Input: part model. Units: mm. Frame: model coordinates. Face numbers are marked on the shaded views. A direction names the side the tool comes from. Coordinates: 2 decimals unless noted, no trailing zeros. Write each loop counter-clockwise with the first axis right and the second up, starting at its lowest first coordinate (ties: lowest second). Pieces come first, ordered by that corner, then holes. Notation, with made-up numbers: (-26, 18.5) - (11, 18.5) arc R14 cw to (11, 45.5) - close; hole circle Ø3 at (-24.75, -27). An arc over 180 degrees is marked (long way). Put each result on its own line as item: value. Start each with the question number.
1. Line query: line 1 (X direction, y = 1.05, z = -11.06); line 2 (Z direction, x = 15.9, y = 0.6); line 3 (Y direction, x = -7, z = -9). Output: solid intervals per line, ascending.
2. Cut plane A-A, the plane z = 0. Return loops of the section in (x, y).
3. Pin query (flat end, axial travel): pin 1 (6.5 mm diameter, centred on x = -19, z = -14.5, fed in from +Y); pin 2 (5.5 mm diameter, centred on x = -17.85, z = 13.01, fed in from -Y); pin 3 (5.5 mm diameter, centred on x = 17.85, z = 13.01, fed in from +Y). Return the tip coordinate at first contact, or that it passes through.
4. Access query for the marked faces 1, 2, 3 and 4. Directions: +Z, -Z, +X, -X, +Y, -Y. A direction counts if a zero-diameter tool reaches every point of the face in a straight line with its end or side. Return the directions, or none.
5. Cut plane C-C, the plane x = 8.5. Return loops of the section in (y, z), and give its area (3 significant figures).
6. Cut plane B-B, the plane y = 5.5. Return loops of the section in (x, z), and give its area (3 significant figures).
from build123d import *

# Parameters (mm, degrees)
CROQUIS1_W              = 41.94
CROQUIS1_H              = 32.26
CROQUIS1_R              = 1.65
CROQUIS1_R_2            = 0.2
SALIENTE_EXTRUIR1_DEPTH = 1.64
CORTAR_EXTRUIR1_START   = -0.1
CROQUIS2_R              = 3.04
CROQUIS2_R_2            = 1.65
CORTAR_EXTRUIR1_DEPTH   = 0.1
REDONDEO2_R             = 3
CROQUIS3_W              = 7.8
CROQUIS3_H              = 10.08
SALIENTE_EXTRUIR2_DEPTH = 6.7


with BuildPart() as part:
    # Croquis1 → Saliente-Extruir1 (new body)
    with BuildSketch(Plane(origin=(0, 0, 0), x_dir=(1, 0, 0), z_dir=(0, 1, 0))):
        Rectangle(CROQUIS1_W, CROQUIS1_H)
        with Locations(Location((-17.85, 13.01, 0), (0, 0, 270))):
            Circle(CROQUIS1_R, mode=Mode.SUBTRACT)
        with Locations(Location((17.85, 13.01, 0), (0, 0, 90))):
            Circle(CROQUIS1_R, mode=Mode.SUBTRACT)
        with Locations(Location((17.85, -13.01, 0), (0, 0, 270))):
            Circle(CROQUIS1_R, mode=Mode.SUBTRACT)
        with Locations(Location((-17.85, -13.01, 0), (0, 0, 90))):
            Circle(CROQUIS1_R, mode=Mode.SUBTRACT)
        with Locations(Location((-15.9, 13.01, 0), (0, 0, 270))):
            Circle(CROQUIS1_R_2, mode=Mode.SUBTRACT)
        with Locations(Location((-16.471141777, 11.631141777, 0), (0, 0, 270))):
            Circle(CROQUIS1_R_2, mode=Mode.SUBTRACT)
        with Locations(Location((-17.85, 11.06, 0), (0, 0, 270))):
            Circle(CROQUIS1_R_2, mode=Mode.SUBTRACT)
        with Locations(Location((-19.228858223, 11.631141777, 0), (0, 0, 270))):
            Circle(CROQUIS1_R_2, mode=Mode.SUBTRACT)
        with Locations(Location((-19.8, 13.01, 0), (0, 0, 270))):
            Circle(CROQUIS1_R_2, mode=Mode.SUBTRACT)
        with Locations(Location((-19.228858223, 14.388858223, 0), (0, 0, 270))):
            Circle(CROQUIS1_R_2, mode=Mode.SUBTRACT)
        with Locations(Location((-17.85, 14.96, 0), (0, 0, 270))):
            Circle(CROQUIS1_R_2, mode=Mode.SUBTRACT)
        with Locations(Location((-16.471141777, 14.388858223, 0), (0, 0, 270))):
            Circle(CROQUIS1_R_2, mode=Mode.SUBTRACT)
        with Locations(Location((19.8, 13.01, 0), (0, 0, 90))):
            Circle(CROQUIS1_R_2, mode=Mode.SUBTRACT)
        with Locations(Location((19.228858223, 14.388858223, 0), (0, 0, 90))):
            Circle(CROQUIS1_R_2, mode=Mode.SUBTRACT)
        with Locations(Location((17.85, 14.96, 0), (0, 0, 90))):
            Circle(CROQUIS1_R_2, mode=Mode.SUBTRACT)
        with Locations(Location((16.471141777, 14.388858223, 0), (0, 0, 90))):
            Circle(CROQUIS1_R_2, mode=Mode.SUBTRACT)
        with Locations(Location((15.9, 13.01, 0), (0, 0, 90))):
            Circle(CROQUIS1_R_2, mode=Mode.SUBTRACT)
        with Locations(Location((16.471141777, 11.631141777, 0), (0, 0, 90))):
            Circle(CROQUIS1_R_2, mode=Mode.SUBTRACT)
        with Locations(Location((19.228858223, 11.631141777, 0), (0, 0, 90))):
            Circle(CROQUIS1_R_2, mode=Mode.SUBTRACT)
        with Locations(Location((17.85, 11.06, 0), (0, 0, 90))):
            Circle(CROQUIS1_R_2, mode=Mode.SUBTRACT)
        with Locations(Location((19.228858223, -11.631141777, 0), (0, 0, 270))):
            Circle(CROQUIS1_R_2, mode=Mode.SUBTRACT)
        with Locations(Location((19.8, -13.01, 0), (0, 0, 270))):
            Circle(CROQUIS1_R_2, mode=Mode.SUBTRACT)
        with Locations(Location((19.228858223, -14.388858223, 0), (0, 0, 270))):
            Circle(CROQUIS1_R_2, mode=Mode.SUBTRACT)
        with Locations(Location((17.85, -14.96, 0), (0, 0, 270))):
            Circle(CROQUIS1_R_2, mode=Mode.SUBTRACT)
        with Locations(Location((16.471141777, -14.388858223, 0), (0, 0, 270))):
            Circle(CROQUIS1_R_2, mode=Mode.SUBTRACT)
        with Locations(Location((15.9, -13.01, 0), (0, 0, 270))):
            Circle(CROQUIS1_R_2, mode=Mode.SUBTRACT)
        with Locations(Location((17.85, -11.06, 0), (0, 0, 270))):
            Circle(CROQUIS1_R_2, mode=Mode.SUBTRACT)
        with Locations(Location((16.471141777, -11.631141777, 0), (0, 0, 270))):
            Circle(CROQUIS1_R_2, mode=Mode.SUBTRACT)
        with Locations(Location((-19.228858223, -14.388858223, 0), (0, 0, 90))):
            Circle(CROQUIS1_R_2, mode=Mode.SUBTRACT)
        with Locations(Location((-17.85, -14.96, 0), (0, 0, 90))):
            Circle(CROQUIS1_R_2, mode=Mode.SUBTRACT)
        with Locations(Location((-16.471141777, -14.388858223, 0), (0, 0, 90))):
            Circle(CROQUIS1_R_2, mode=Mode.SUBTRACT)
        with Locations(Location((-15.9, -13.01, 0), (0, 0, 90))):
            Circle(CROQUIS1_R_2, mode=Mode.SUBTRACT)
        with Locations(Location((-19.8, -13.01, 0), (0, 0, 90))):
            Circle(CROQUIS1_R_2, mode=Mode.SUBTRACT)
        with Locations(Location((-19.228858223, -11.631141777, 0), (0, 0, 90))):
            Circle(CROQUIS1_R_2, mode=Mode.SUBTRACT)
        with Locations(Location((-17.85, -11.06, 0), (0, 0, 90))):
            Circle(CROQUIS1_R_2, mode=Mode.SUBTRACT)
        with Locations(Location((-16.471141777, -11.631141777, 0), (0, 0, 90))):
            Circle(CROQUIS1_R_2, mode=Mode.SUBTRACT)
    extrude(amount=SALIENTE_EXTRUIR1_DEPTH)

    # Croquis2 → Cortar-Extruir1 (cut)
    # profile 1 of 4: a face of its own
    with BuildSketch(Plane(origin=(0, 1.64, 0), x_dir=(1, 0, 0), z_dir=(0, 1, 0)).offset(CORTAR_EXTRUIR1_START)):
        with Locations(Location((-17.85, 13.01, 0), (0, 0, 270))):
            Circle(CROQUIS2_R)
        with Locations(Location((-17.85, 13.01, 0), (0, 0, 270))):
            Circle(CROQUIS2_R_2, mode=Mode.SUBTRACT)
    # profile 2 of 4: a face of its own
    with BuildSketch(Plane(origin=(0, 1.64, 0), x_dir=(1, 0, 0), z_dir=(0, 1, 0)).offset(CORTAR_EXTRUIR1_START)):
        with Locations(Location((17.85, 13.01, 0), (0, 0, 90))):
            Circle(CROQUIS2_R)
        with Locations(Location((17.85, 13.01, 0), (0, 0, 90))):
            Circle(CROQUIS2_R_2, mode=Mode.SUBTRACT)
    # profile 3 of 4: a face of its own
    with BuildSketch(Plane(origin=(0, 1.64, 0), x_dir=(1, 0, 0), z_dir=(0, 1, 0)).offset(CORTAR_EXTRUIR1_START)):
        with Locations(Location((17.85, -13.01, 0), (0, 0, 270))):
            Circle(CROQUIS2_R)
        with Locations(Location((17.85, -13.01, 0), (0, 0, 270))):
            Circle(CROQUIS2_R_2, mode=Mode.SUBTRACT)
    # profile 4 of 4: a face of its own
    with BuildSketch(Plane(origin=(0, 1.64, 0), x_dir=(1, 0, 0), z_dir=(0, 1, 0)).offset(CORTAR_EXTRUIR1_START)):
        with Locations(Location((-17.85, -13.01, 0), (0, 0, 90))):
            Circle(CROQUIS2_R)
        with Locations(Location((-17.85, -13.01, 0), (0, 0, 90))):
            Circle(CROQUIS2_R_2, mode=Mode.SUBTRACT)
    extrude(amount=CORTAR_EXTRUIR1_DEPTH, mode=Mode.SUBTRACT)

    # Redondeo2
    redondeo2_edges = [part.edges().sort_by_distance(p)[0] for p in [
        (20.97, 0.82, 16.13),
        (-20.97, 0.82, 16.13),
        (-20.97, 0.82, -16.13),
        (20.97, 0.82, -16.13),
    ]]
    fillet(redondeo2_edges, radius=REDONDEO2_R)

    # Croquis3 → Saliente-Extruir2 (add)
    with BuildSketch(Plane(origin=(0, 1.64, 0), x_dir=(1, 0, 0), z_dir=(0, 1, 0))):
        with Locations((17.07, -0.29)):
            Rectangle(CROQUIS3_W, CROQUIS3_H)
    extrude(amount=SALIENTE_EXTRUIR2_DEPTH)


solid = part.part
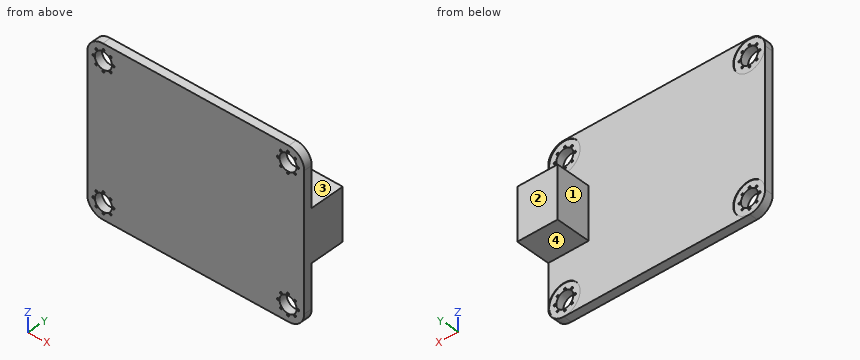
Report:
1. line 1: x = -20.97 to -18.05, -17.65 to 17.65, 18.05 to 20.97
1. line 2: z = -16.13 to -13.21, -12.81 to 12.81, 13.21 to 16.13
1. line 3: y = 0 to 1.64
2. outline: (-20.97, 0) - (20.97, 0) - (20.97, 8.34) - (13.17, 8.34) - (13.17, 1.64) - (-20.97, 1.64) - close
3. pin 1: stops at y = 1.64
3. pin 2: stops at y = 0
3. pin 3: stops at y = 1.54
4. face 1: +Z, -Z, -X, +Y
4. face 2: +Z, -Z, +X, -X, +Y
4. face 3: +Z, +X, -X, +Y
4. face 4: -Z, +X, -X, +Y
5. outline: (0, -16.13) - (1.64, -16.13) - (1.64, 16.13) - (0, 16.13) - close
5. area: 52.9 mm^2
6. outline: (13.17, -4.75) - (20.97, -4.75) - (20.97, 5.33) - (13.17, 5.33) - close
6. area: 78.6 mm^2
